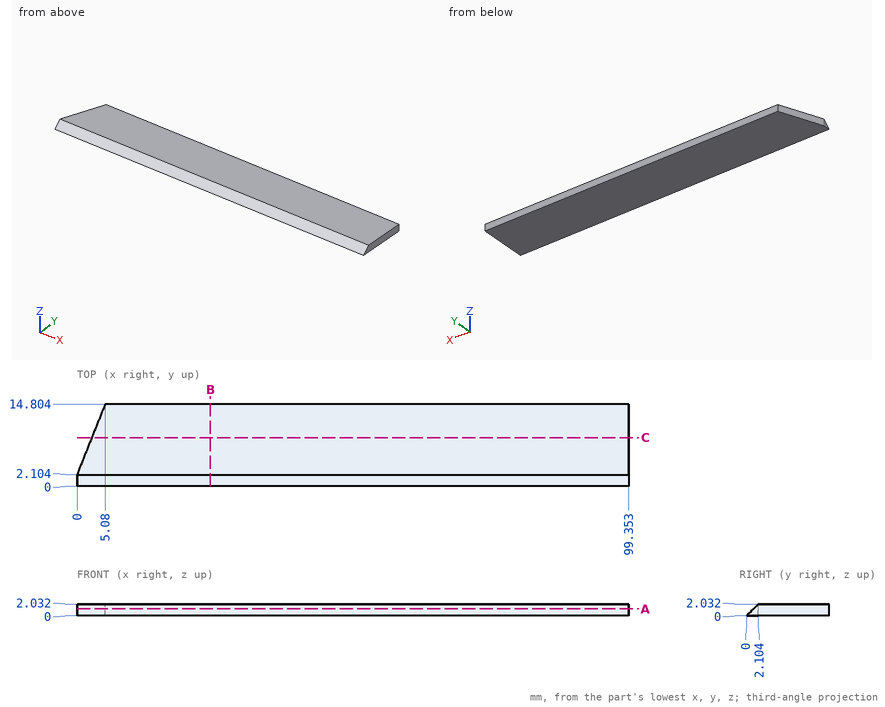
Design review of the part shown in the three views and the two pictorial views. Dimensions are in mm from the part's minimum x, y and z. Coordinates: 2 decimals unless noted, no trailing zeros. Order: outer loops, then holes, each group sorted by start corner. A loop starts at its lowest first (then second) coordinate and runs counter-clockwise, first axis right, second up. Notation, with made-up numbers: (41, 58) - (72, 58) arc R37 ccw to (72, 97) - close; hole circle Ø10 at (60, 57). An arc over 180 degrees is marked (long way). One line per question, with ' | ' between items.
Q1. To check wall thickness, follow line 1 along Y through (x, z) = (88, 1.95) (1 decimal); line 2 along X through (y, z) = (12.25, 1.85); line 3 along X through (y, z) = (5.5, 0.2). State the ranges of each line that lie inside material, in increasing order.
Answer key:
line 1: y = 2 to 14.8 | line 2: x = 4.06 to 99.35 | line 3: x = 1.36 to 99.35
Q2. Consider section B-B, the plane x = 24. Give the boundary of the cut face in (y, z).
Answer key:
outline: (0, 0) - (14.8, 0) - (14.8, 2.03) - (2.1, 2.03) - close
Q3. Consider section A-A, the plane z = 1.2. Give the boundary of the cut face in (x, y).
Answer key:
outline: (0, 1.24) - (99.35, 1.24) - (99.35, 14.8) - (5.08, 14.8) - (0, 2.1) - close
Q4. Consider section C-C, the plane y = 8.75. Give the boundary of the cut face in (x, z).
Answer key:
outline: (2.66, 0) - (99.35, 0) - (99.35, 2.03) - (2.66, 2.03) - close
